The model under review builds one solid part; all positions refer to its coordinate system, in mm. Face numbers are marked on the shaded views. A direction names the side the tool comes from. Coordinates: 2 decimals unless noted, no trailing zeros. Write each loop counter-clockwise with the first axis right and the second up, starting at its lowest first coordinate (ties: lowest second). Pieces come first, ordered by that corner, then holes. Notation, with made-up numbers: (54, 61) - (86, 61) arc R30 cw to (86, 98) - close; hole circle Ø8 at (8, 66.25). An arc over 180 degrees is marked (long way). Put each result on its own line as item: value.
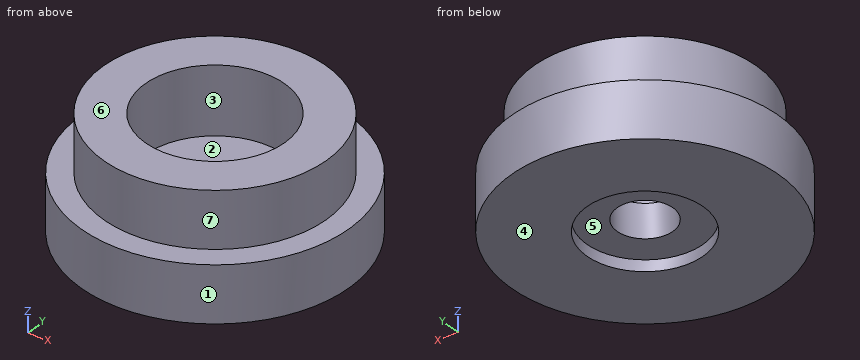
from build123d import *

# Parameters (mm, degrees)
SKETCH_2_R          = 20
EXTRUDE_1_DEPTH     = 10
SKETCH_3_R          = 5
CUT_EXTRUDE_1_DEPTH = 21
SKETCH_4_R          = 12.5
CUT_EXTRUDE_2_DEPTH = 12


with BuildPart() as part:
    # 草图1 → 旋转1 (revolve)
    with BuildSketch(Plane(origin=(0, 0, 0), x_dir=(0, 0, -1), z_dir=(1, 0, 0))):
        Polygon((0, 0), (0, 24), (10, 24), (10, 10.45), (8, 10.45), (8, 0), align=None)
    revolve(axis=Axis((0, 0, 0), (0, 0, -1)))

    # 草图2 → 凸台-拉伸1 (add)
    with BuildSketch(Plane.XY):
        Circle(SKETCH_2_R)
    extrude(amount=EXTRUDE_1_DEPTH)

    # 草图3 → 切除-拉伸1 (cut, through all)
    with BuildSketch(Plane.XY.offset(10)):
        Circle(SKETCH_3_R)
    extrude(amount=-CUT_EXTRUDE_1_DEPTH, mode=Mode.SUBTRACT)

    # 草图4 → 切除-拉伸2 (cut)
    with BuildSketch(Plane.XY.offset(10)):
        Circle(SKETCH_4_R)
    extrude(amount=-CUT_EXTRUDE_2_DEPTH, mode=Mode.SUBTRACT)


solid = part.part
1. Machinability: for the marked faces 5, 6 and 7, which of the approach directions +Z, -Z, +X, -X, +Y, -Y give a long, thin tool a straight path to every point of the face, cutting with its end or side? Answer none if there is none.
Determined:
face 5: -Z
face 6: +Z, +X, -X, +Y, -Y
face 7: +Z
2. Consider section A-A on y = 0. State the section outline as (x, z) points.
Determined:
outline: (-24, -10) - (-10.45, -10) - (-10.45, -8) - (-5, -8) - (-5, -2) - (-12.5, -2) - (-12.5, 10) - (-20, 10) - (-20, 0) - (-24, 0) - close; (5, -8) - (10.45, -8) - (10.45, -10) - (24, -10) - (24, 0) - (20, 0) - (20, 10) - (12.5, 10) - (12.5, -2) - (5, -2) - close
3. The part is to be moulded in two halves that separate along X. For the marked faces 1, 2, 3 and 4, say which applies: +X half, -X half, draft (parallel to the pull), parting line (faces both ways), or undercut.
Determined:
face 1: parting line
face 2: undercut
face 3: undercut
face 4: draft
4. Consider section D-D on z = 7.5. State the section outline as (x, y) points.
Determined:
outline: circle Ø40 at (0, 0); hole circle Ø25 at (0, 0)
5. For pin 1 Ø5 at (y, z) = (10, -1) entering from -X; pin 2 Ø3 at (y, z) = (-17, 3) entering from -X; pin 3 Ø2 at (y, z) = (-1.5, 8) entering from +X, all flat-tipped, find the tip position at first contact; note any pin that passes through.
Determined:
pin 1: stops at x = -22.8
pin 2: stops at x = -12.64
pin 3: stops at x = 19.99
6. To check wall thickness, follow probe 1 along Y at (x, z) = (0, 5.75); probe 2 along Z at (x, y) = (6, -4.5); probe 3 along Y at (x, z) = (-8.5, 6.5). State the ranges of each line that lie inside material, in increasing order.
Determined:
probe 1: y = -20 to -12.5, 12.5 to 20
probe 2: z = -8 to -2
probe 3: y = -18.1 to -9.17, 9.17 to 18.1
7. Consider section C-C on y = -18. State the section outline as (x, z) points.
Determined:
outline: (-15.87, -10) - (15.87, -10) - (15.87, 0) - (8.72, 0) - (8.72, 10) - (-8.72, 10) - (-8.72, 0) - (-15.87, 0) - close
